The listing builds one solid part. Answer for the finished solid, in the listing's coordinates (mm). Face numbers are marked on the shaded views. A direction names the side the tool comes from. Round coordinates to 2 decimals unless told otherwise and drop trailing zeros. Write each loop counter-clockwise with the first axis right and the second up, starting at its lowest first coordinate (ties: lowest second). Pieces come first, ordered by that corner, then holes. Notation, with made-up numbers: M -27,80 L -8,80 A26 ccw -8,98 Z; hole C 78.25,43 d2. An arc over 180 degrees is marked long. One line per item, written item: value. Start each with the question number.
(1) Section A-A (y = 0) is taken. Determine the outline of the cut face in (x, z), plus the area to 3 significant figures.
(2) Given P1, Ø1.5, axis at x = 4, y = -6.5, coming from the +Z side; P2, Ø1.5, axis at y = 2, z = 2, coming from the +X side; P3, Ø5, axis at x = 4.24, y = 4.24, coming from the +Z side, each flat-ended and moving along its own axis, determine where each tip first touches the part or whether it passes through.
(3) Consider probe 1 along X at (y, z) = (6.75, 1.85); probe 2 along Y at (x, z) = (-6, 1.1); probe 3 along Y at (x, z) = (0, 3.15). Determine where each line is inside the solid, lowest interval first.
(4) Section D-D (x = -5.5) is taken. State how many separate pieces and enclosed holes the cut face has, plus the area to 3 significant figures.
(5) Section C-C (z = 3.2) is taken. Determine the outline of the cut face in (x, y).
(6) For the marked faces 1 and 2, determine the directions among +Z, -Z, +X, -X, +Y, -Y from which every point of the face is accessible in a straight line to the end or side of a thin tool.
(7) For a pull along X with two mould halves and no side action, classify the marked faces 3, 4 and 5 as released by +X, released by -X, zero draft, split by the parting line, or undercut.
```python
from build123d import *

# Parameters (mm, degrees)
SKETCH1_R           = 9
SKETCH1_R_2         = 1.55
BOSS_EXTRUDE1_DEPTH = 2
SKETCH2_R           = 3
BOSS_EXTRUDE2_DEPTH = 1.5
SKETCH3_R           = 2.5
BOSS_EXTRUDE3_DEPTH = 2.4
CHAMFER1_SIZE       = 1.4


with BuildPart() as part:
    # Sketch1 → Boss-Extrude1 (new body)
    with BuildSketch(Plane(origin=(0, 0, 0), x_dir=(0, 1, 0), z_dir=(0, 0, 1))):
        with Locations(Location((0, 0, 0), (0, 0, 270))):
            Circle(SKETCH1_R)
        with Locations(Location((-4.242640687, 4.242640687, 0), (0, 0, 270))):
            Circle(SKETCH1_R_2, mode=Mode.SUBTRACT)
        with Locations(Location((4.242640687, 4.242640687, 0), (0, 0, 270))):
            Circle(SKETCH1_R_2, mode=Mode.SUBTRACT)
        with Locations(Location((4.242640687, -4.242640687, 0), (0, 0, 270))):
            Circle(SKETCH1_R_2, mode=Mode.SUBTRACT)
        with Locations(Location((-4.242640687, -4.242640687, 0), (0, 0, 270))):
            Circle(SKETCH1_R_2, mode=Mode.SUBTRACT)
    extrude(amount=BOSS_EXTRUDE1_DEPTH)

    # Sketch2 → Boss-Extrude2 (add)
    with BuildSketch(Plane.XY.offset(2)):
        Circle(SKETCH2_R)
    extrude(amount=BOSS_EXTRUDE2_DEPTH)

    # Sketch3 → Boss-Extrude3 (add)
    with BuildSketch(Plane.XY.offset(3.5)):
        Circle(SKETCH3_R)
    extrude(amount=BOSS_EXTRUDE3_DEPTH)

    # Chamfer1
    chamfer1_edges = [part.edges().sort_by_distance(p)[0] for p in [
        (2.692640687, 4.242640687, 2),
        (2.692640687, -4.242640687, 2),
        (-5.792640687, 4.242640687, 2),
        (-5.792640687, -4.242640687, 2),
    ]]
    chamfer(chamfer1_edges, length=CHAMFER1_SIZE)


solid = part.part
```
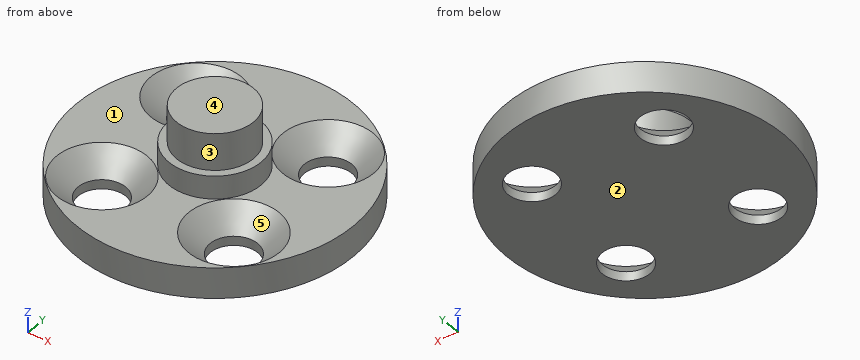
Recorded:
1. outline: M -9,0 L 9,0 L 9,2 L 3,2 L 3,3.5 L 2.5,3.5 L 2.5,5.9 L -2.5,5.9 L -2.5,3.5 L -3,3.5 L -3,2 L -9,2 Z
1. area: 57.0 mm2
2. P1: stops at z = 2
2. P2: stops at x = 8.91
2. P3: stops at z = 1.55
3. probe 1: x = -5.95 to -5.49, -3 to 3, 5.49 to 5.95
3. probe 2: y = -6.71 to -5.3, -3.19 to 3.19, 5.3 to 6.71
3. probe 3: y = -3 to 3
4. separate pieces: 3
4. enclosed holes: 0
4. area: 16.0 mm2
5. outline: C 0,0 d6
6. face 1: +Z
6. face 2: -Z, +X, -X, +Y, -Y
7. face 3: split by the parting line
7. face 4: zero draft
7. face 5: undercut
